Could you check a few things on this model? Use its own coordinates, in mm. A direction names the side the tool comes from. Give positions to 0.01 mm unless a question says otherwise; leave off trailing zeros. Write each loop counter-clockwise with the first axis right and the second up, starting at its lowest first coordinate (ties: lowest second). Pieces come first, ordered by that corner, then holes. Notation, with made-up numbers: M 84.5,-5.75 L 107.5,-5.75 A26 ccw 107.5,15.25 Z; hole C 40,-28 d3. An arc over 180 degrees is marked long. Answer as CSV lines item,"result". Start each with the question number.
from build123d import *

# Parameters (mm, degrees)
SKETCH_1_R          = 1.5
EXTRUDE_1_DEPTH     = 8
SKETCH_2_R          = 2.5
CUT_EXTRUDE_1_DEPTH = 4


with BuildPart() as part:
    # 草图1 → 凸台-拉伸1 (new body)
    with BuildSketch(Plane.XY):
        with BuildLine():
            Line((26.30677697, 11), (26.30677697, 0))
            ThreePointArc((26.30677697, 0), (25.231575927, -1.895238991), (24.29677697, -3.863522261))
            Line((24.29677697, -3.863522261), (11.30677697, -5))
            Line((11.30677697, -5), (11.30677697, 11))
            Line((11.30677697, 11), (26.30677697, 11))
        make_face()
        with Locations((19.467365682, 3.704627959)):
            Circle(SKETCH_1_R, mode=Mode.SUBTRACT)
    extrude(amount=EXTRUDE_1_DEPTH)

    # 草图2 → 切除-拉伸1 (cut)
    with BuildSketch(Plane.XY.offset(8)):
        with Locations((19.467365682, 3.704627959)):
            Circle(SKETCH_2_R)
    extrude(amount=-CUT_EXTRUDE_1_DEPTH, mode=Mode.SUBTRACT)


solid = part.part
1. Please list where these lines run through material, in increasing order: line 1 (Z direction, x = 20, y = 6); line 2 (Y direction, x = 20, z = 1); line 3 (Y direction, x = 21.75, z = 6.25).
2. Imagine slicing it at B-B, the plane x = 20. Please give me the cut outline in (y, z), plus the area to 3 significant figures.
3. Imagine slicing it at C-C, the plane z = 4.75. Please give me the cut outline in (x, y).
4. Will this pin go through, and if not, where does the flat tip stop? P1, Ø8, axis at x = 14.5, y = 6, coming from the -Z side.
5. Imagine slicing it at A-A, the plane y = 2.75. Please give me the cut outline in (x, z).
6. On a 3-axis mill with a long thin cutter (end or side, diameter ignored), from which of +Z, -Z, +X, -X, +Y, -Y can I reach the whole of each face in a straight line? I mean faces 1 (the cylindrical face through (16.97, 3.81, 6.03)), 2 (the cylindrical face through (25.246, -1.868, 3.944)). Say none if no direction works.
7. Imagine slicing it at D-D, the plane y = 5.5. Please give me the cut outline in (x, z), plus the area to 3 significant figures.
8. Thinking about a two-plate mould opening in X: for faces 3 (the flat face through (17.893, -4.424, 3.944)), 4 (the flat face through (17, 3, 0)), 5 (the flat face through (21, 3, 4)), which applies, pulls with the +X half, pulls with the -X half, needs draft (parallel to the pull), parting line crosses it, or undercut?
Solutions:
1,line 1,"0 to 4"
1,line 2,"-4.24 to 2.3, 5.11 to 11"
1,line 3,"-4.09 to 2.69, 4.72 to 11"
2,outline,"M -4.24,0 L 2.3,0 L 2.3,4 L 1.26,4 L 1.26,8 L -4.24,8 Z; M 5.11,0 L 11,0 L 11,8 L 6.15,8 L 6.15,4 L 5.11,4 Z"
2,area,"91.2 mm²"
3,outline,"M 11.31,-5 L 24.3,-3.86 A30 cw 26.31,0 L 26.31,11 L 11.31,11 Z; hole C 19.47,3.7 d5"
4,P1,"z = 0"
5,outline,"M 11.31,0 L 18.31,0 L 18.31,4 L 17.16,4 L 17.16,8 L 11.31,8 Z; M 20.62,0 L 26.31,0 L 26.31,8 L 21.78,8 L 21.78,4 L 20.62,4 Z"
6,face 1,"+Z"
6,face 2,"+Z, -Z, +X, -Y"
7,outline,"M 11.31,0 L 26.31,0 L 26.31,8 L 21.21,8 L 21.21,4 L 17.73,4 L 17.73,8 L 11.31,8 Z"
7,area,"106 mm²"
8,face 3,"pulls with the +X half"
8,face 4,"needs draft"
8,face 5,"undercut"
